For this review, take the finished solid that the model builds, in its own axes (mm). A direction names the side the tool comes from. Round coordinates to 2 decimals unless told otherwise and drop trailing zeros. Loops run counter-clockwise (first coordinate to the right, second up) from the corner with the lowest first, then second, coordinate; pieces in that order, holes last. Notation, with made-up numbers: (26, 43) -> (72, 43) arc R30 ccw to (72, 82) -> close; hole circle Ø9 at (26, -4.5). An arc over 180 degrees is marked (long way). One line per question, with ' | ' between items. Start each with the question number.
1. Consider section A-A (x = 1). Write out the cut boundary in (y, z).
2. Consider section B-B (z = 0). Write out the cut boundary in (x, y).
3. For pin 1 Ø3.5 at (x, y) = (-1.5, 7.5) entering from +Z; pin 2 Ø3 at (x, z) = (-2, 13.5) entering from -Y; pin 3 Ø10.5 at (y, z) = (1.5, 3) entering from -X; pin 4 Ø8 at (y, z) = (0, 0) entering from +X, all flat-tipped, find the tip position at first contact; note any pin that passes through.
4. Wall thickness on line 1 along X through (y, z) = (17, -15); line 2 along Z through (x, y) = (-2.5, 0); line 3 along X through (y, z) = (14.9, 15): over which ranges is each line inside the solid? List them lowest first.
5. For faces 1 (the face through (5.25, -5, -2)), 2 (the face through (0, 7, -10)), 3 (the face through (0, 15, -12)), list the 3-axis set-ups (+Z, -Z, +X, -X, +Y, -Y) from which the entire face can be reached by the end or side of a thin tool; tool diameter is ignored.
6. Consider section C-C (x = -3.5). Write out the cut boundary in (y, z), and give its area (3 significant figures).
7. Consider section D-D (z = 15). Write out the cut boundary in (x, y), and give its area (3 significant figures).
8. Draft analysis for pull direction X (two halves, no side actions). For faces 4 (the face through (6.25, 7, 0)), 5 (the face through (0, 18, 0)), 6 (the face through (0, 16, 13)), state which applies: pulls with the +X half, pulls with the -X half, needs draft (parallel to the pull), parting line crosses it, or undercut.
Autodesk Inventor part; units mm, degrees
ref_plane "YZ Plane" through (0, 0, 0) normal (1, 0, 0) x (0, 1, 0)
ref_plane "XZ Plane" through (0, 0, 0) normal (0, 1, 0) x (-1, 0, 0)
ref_plane "XY Plane" through (0, 0, 0) normal (0, 0, 1) x (1, 0, 0)
sketch "Sketch1" plane through (0, 0, 0) normal (1, 0, 0) x (0, 1, 0)
  line L0 (0, 0) -> (14, 0) construction
  line L1 (0, -10) -> (14, -10)
  line L2 (14, 10) -> (0, 10)
  arc A0 (0, 10) -> (0, -10) centre (0, 0) ccw
  arc A1 (14, -10) -> (14, 10) centre (14, 0) ccw construction
  line L3 (14, 10) -> (14, -10)
  point P0 (7, 0)
  dimension "d2" = 20
  dimension "d1" = 14
extrude "Extrusion1" add sketch "Sketch1" along normal mid plane 10.5
sketch "Sketch2" plane through (-5.25, 14, 10) normal (0, 1, 0) x (1, 0, 0)
  line L0 (0, -10) -> (10.5, -10)
  line L1 (10.5, -10) -> (10.5, 30)
  line L2 (10.5, 30) -> (0, 30)
  line L3 (0, 30) -> (0, -10)
  line L4 (0, 0) -> (0, 20) construction
  line L5 (0, 20) -> (10.5, 20) construction
  line L6 (10.5, 20) -> (10.5, 0) construction
  line L7 (10.5, 0) -> (0, 0) construction
  line L8 (0, 0) -> (0, 20) construction
  line L9 (10.5, 20) -> (10.5, 0) construction
  line L10 (0, 10) -> (10.5, 10) construction
  point P0 (5.25, 10)
  dimension "d28" = 40
extrude "Extrusion2" add sketch "Sketch2" along normal blind 4
sketch "Sketch3" plane through (-5.25, 14, 10) normal (0, -1, 0) x (1, 0, 0)
  line L0 (10.5, -30) -> (0, -30)
  line L1 (0, -30) -> (0, -20)
  line L2 (0, -20) -> (0, 0)
  line L3 (0, 0) -> (0, 10)
  line L4 (0, 10) -> (10.5, 10)
  line L5 (10.5, 10) -> (10.5, 0)
  line L6 (10.5, 0) -> (10.5, -20)
  line L7 (10.5, -20) -> (10.5, -30)
  line L8 (10.5, -20) -> (0, -20)
  line L9 (0, 0) -> (10.5, 0)
  line L10 (0, 10) -> (10.5, 10)
  point P0 (5.25, -10)
  point P1 (5.25, 5)
  point P2 (5.25, -25)
  point P3 (5.25, 10)
  point P4 (5.25, 10)
  point P5 (5.25, 10)
  dimension "d30" = 5
  dimension "d31" = 5
hole "Hole1" at (0, 14, 15) at (0, 14, -15) direction (0, 1, 0) diameter 3.4 end through all counterbore diameter 6 counterbore depth 2
sketch "Sketch5" plane through (5.25, 0, 0) normal (1, 0, 0) x (0, 0, -1)
  arc A0 (-10, 0) -> (10, 0) centre (0, 0) ccw
hole "Hole3" at (5.25, 0, 0) direction (-1, 0, 0) diameter 13 end through all
thicken "Thicken1" operation add thickness 0.15 both sides no extend neighbours yes toward (0, 0.0804666, -0.9967573) faces at (1.75, 0.523, -6.4789)
sketch "Sketch6" plane through (5.25, 0, 0) normal (1, 0, 0) x (0, 0, -1)
  circle A0 centre (0, 0) radius 6.65 construction
  line L0 (20, 18) -> (20, 14)
  line L1 (20, 14) -> (10, 14)
  line L2 (10, 14) -> (10, 0)
  arc A1 (-10, 0) -> (10, 0) centre (0, 0) ccw
  line L3 (-10, 0) -> (-10, 14)
  line L4 (-10, 14) -> (-20, 14)
  line L5 (-20, 14) -> (-20, 18)
  line L6 (-20, 18) -> (20, 18)
  circle A2 centre (0, 0) radius 6.65
  line L7 (20, 18) -> (20, 14)
  line L8 (20, 14) -> (10, 14)
  line L9 (10, 14) -> (10, 0)
  arc A3 (-10, 0) -> (10, 0) centre (0, 0) ccw
  line L10 (-10, 0) -> (-10, 14)
  line L11 (-10, 14) -> (-20, 14)
  line L12 (-20, 14) -> (-20, 18)
  line L13 (-20, 18) -> (20, 18)
  circle A4 centre (0, 0) radius 5.15
  dimension "d37" = 1.5
extrude "Extrusion3" add sketch "Sketch6" along normal blind 1 contours L0 L1 L2 A1 L3 L4 L5 L6 | A2
chamfer "Chamfer2" distance 0.5 angle 45 1 edges at (-5.25, 0, 6.65)
chamfer "Chamfer3" distance 1 angle 45 1 edges at (6.25, 18, 0)
equation "\"d21\" = diameter"
equation "\"diameter\" = 13"
properties part number "bearing holder"
Answer block:
1) outline: (0, -10) -> (14, -10) -> (14, -12.17) -> (16, -12.17) -> (16, -13.63) -> (18, -13.63) -> (18, 13.63) -> (16, 13.63) -> (16, 12.17) -> (14, 12.17) -> (14, 10) -> (0, 10) arc R10 ccw to start; (14, -20) -> (18, -20) -> (18, -16.37) -> (16, -16.37) -> (16, -17.83) -> (14, -17.83) -> close; (14, 17.83) -> (16, 17.83) -> (16, 16.37) -> (18, 16.37) -> (18, 20) -> (14, 20) -> close; hole circle Ø13.3 at (0, 0)
2) outline: (-5.25, -10) -> (6.25, -10) -> (6.25, -5.15) -> (5.25, -5.15) -> (5.25, -6.65) -> (-4.75, -6.65) -> (-5.25, -7.15) -> close; (-5.25, 7.15) -> (-4.75, 6.65) -> (5.25, 6.65) -> (5.25, 5.15) -> (6.25, 5.15) -> (6.25, 17) -> (5.25, 18) -> (-5.25, 18) -> close
3) pin 1: stops at z = 10 | pin 2: stops at y = 14 | pin 3: stops at x = -5.25 | pin 4: passes through
4) line 1: x = -5.25 to -1.7, 1.7 to 6.25 | line 2: z = -10 to -6.65, 6.65 to 10 | line 3: x = -5.25 to -3, 3 to 6.25
5) face 1: -X | face 2: -Z, +X, -X, -Y | face 3: -Y
6) outline: (0, -10) -> (14, -10) -> (14, -20) -> (18, -20) -> (18, 20) -> (14, 20) -> (14, 10) -> (0, 10) arc R10 ccw to start; hole circle Ø13.3 at (0, 0) | area: 458 mm2
7) outline: (-5.25, 14) -> (-3, 14) -> (-3, 16) -> (-1.7, 16) -> (-1.7, 18) -> (-5.25, 18) -> close; (1.7, 16) -> (3, 16) -> (3, 14) -> (6.25, 14) -> (6.25, 17) -> (5.25, 18) -> (1.7, 18) -> close | area: 26.7 mm2
8) face 4: pulls with the +X half | face 5: needs draft | face 6: undercut
